```python
from build123d import *

# Parameters (mm, degrees)
F0_R     = 100
F0_R_2   = 20
F0_R_3   = 44.95
F0_R_4   = 44.45
F1_DEPTH = 50
F2_SIZE  = 4


with BuildPart() as f1:
    # F0 (on Top) → F1 (new body)
    with BuildSketch(Plane.XY):
        Circle(F0_R)
        with Locations((0, -65)):
            Circle(F0_R_2, mode=Mode.SUBTRACT)
        with Locations((-50, 0)):
            Circle(F0_R_3, mode=Mode.SUBTRACT)
        with Locations((50, 0)):
            Circle(F0_R_4, mode=Mode.SUBTRACT)
    extrude(amount=F1_DEPTH)

    # F2
    f2_edges = [f1.edges().sort_by_distance(p)[0] for p in [
        (5.55, 0, 50),
        (-94.95, 0, 50),
        (-20, -65, 50),
        (5.55, 0, 0),
        (-94.95, 0, 0),
        (-20, -65, 0),
    ]]
    chamfer(f2_edges, length=F2_SIZE)


solid = f1.part
```
The listing builds one solid part. Answer for the finished solid, in the listing's coordinates (mm). Give positions to 0.01 mm unless a question says otherwise; leave off trailing zeros. Order: outer loops, then holes, each group sorted by start corner. A loop starts at its lowest first (then second) coordinate and runs counter-clockwise, first axis right, second up.
Item 1: The part is cut by section C-C, the plane z = 17.5. Give the vertices of the cut face in (x, y), and give its area (3 significant figures).
From the geometry:
outline: circle Ø200 at (0, 0); hole circle Ø89.9 at (-50, 0); hole circle Ø40 at (0, -65); hole circle Ø88.9 at (50, 0)
area: 17,600 mm2
Item 2: For a pull along Y with two mould halves and no side action, classify faces 1 (the face through (0, 0, 0)), 2 (the face through (92.397, 13.352, 24.706)), 3 (the face through (95.38, 30.04, 24.65)) as pulls with the +Y half, pulls with the -Y half, needs draft (parallel to the pull), parting line crosses it, or undercut.
From the geometry:
face 1: needs draft
face 2: undercut
face 3: parting line crosses it
Item 3: The part is cut by section B-B, the plane x = -50. Give the vertices of the cut face in (y, z), and give its area (3 significant figures).
From the geometry:
outline: (-86.6, 0) - (-48.95, 0) - (-44.95, 4) - (-44.95, 46) - (-48.95, 50) - (-86.6, 50) - close; (44.95, 4) - (48.95, 0) - (86.6, 0) - (86.6, 50) - (48.95, 50) - (44.95, 46) - close
area: 4,130 mm2
Item 4: Find the intervals of material crossed by probe 1 along Y at (x, z) = (18, 23); probe 2 along X at (y, z) = (4, 4); probe 3 along Y at (x, z) = (-10, 3), in increasing order.
From the geometry:
probe 1: y = -98.37 to -73.72, -56.28 to -30.85, 30.85 to 98.37
probe 2: x = -99.92 to -94.77, -5.23 to 5.73, 94.27 to 99.92
probe 3: y = -99.5 to -83.47, -46.53 to -22.61, 22.61 to 99.5
Item 5: Given pin 1 Ø12 at (x, z) = (69, 5) entering from +Y; pin 2 Ø1 at (x, z) = (-34, 24) entering from +Y; pin 3 Ø1.5 at (y, z) = (65, 36.5) entering from +X, each flat-ended and moving along its own axis, determine where each tip first touches the part or whether it passes through.
From the geometry:
pin 1: stops at y = 77.66
pin 2: stops at y = 94.22
pin 3: stops at x = 76.63
Item 6: The part is cut by section D-D, the plane y = -65. Give the vertices of the cut face in (x, z), and give its area (3 significant figures).
From the geometry:
outline: (-75.99, 0) - (-24, 0) - (-20, 4) - (-20, 46) - (-24, 50) - (-75.99, 50) - close; (20, 4) - (24, 0) - (75.99, 0) - (75.99, 50) - (24, 50) - (20, 46) - close
area: 5,570 mm2
Item 7: The part is cut by section A-A, the plane y = 0. Give the vertices of the cut face in (x, z), and give its area (3 significant figures).
From the geometry:
outline: (-100, 0) - (-98.95, 0) - (-94.95, 4) - (-94.95, 46) - (-98.95, 50) - (-100, 50) - close; (-5.05, 4) - (-1.05, 0) - (1.55, 0) - (5.55, 4) - (5.55, 46) - (1.55, 50) - (-1.05, 50) - (-5.05, 46) - close; (94.45, 4) - (98.45, 0) - (100, 0) - (100, 50) - (98.45, 50) - (94.45, 46) - close
area: 996 mm2
